from build123d import *

# Parameters (mm, degrees)
F1_DEPTH = 19.05
F2_R     = 76.2
F3_R     = 50.8
F4_R     = 8.994508
F5_DEPTH = 25.4


with BuildPart() as f1:
    # F0 (on Front) → F1 (new body)
    with BuildSketch(Plane.XZ):
        Polygon((-342.9, 69.85), (-342.9, 0), (266.7, 0), (266.7, 69.85), (139.7, 69.85), (58.081341, 127), (-58.081341, 127), (-139.7, 69.85), align=None)
    extrude(amount=F1_DEPTH)

    # F2
    f2_edges = [f1.edges().sort_by_distance(p)[0] for p in [
        (139.7, -9.525, 69.85),
        (58.081341, -9.525, 127),
        (-58.081341, -9.525, 127),
        (-139.7, -9.525, 69.85),
    ]]
    fillet(f2_edges, radius=F2_R)

    # F3
    f3_edges = [f1.edges().sort_by_distance(p)[0] for p in [
        (266.7, -9.525, 69.85),
        (-342.9, -9.525, 69.85),
    ]]
    fillet(f3_edges, radius=F3_R)

    # F4 (on face) → F5 (cut)
    with BuildSketch(Plane.XZ.offset(19.05)):
        with Locations((-292.1, 37.072986)):
            Circle(F4_R)
    extrude(amount=-F5_DEPTH, mode=Mode.SUBTRACT)


solid = f1.part
The model under review builds one solid part; all positions refer to its coordinate system, in mm. A direction names the side the tool comes from. Round coordinates to 2 decimals unless told otherwise and drop trailing zeros. Loops run counter-clockwise (first coordinate to the right, second up) from the corner with the lowest first, then second, coordinate; pieces in that order, holes last. Notation, with made-up numbers: (-6, 21) -> (28, 21) arc R10 cw to (28, 39) -> close; hole circle Ø3 at (-3.75, 79). An arc over 180 degrees is marked (long way). Write item = value, one per line. Start each with the question number.
Item 1: To check wall thickness, follow L1, parallel to Z at x = -292.1, y = -8.25; L2, parallel to Z at x = -178.5, y = -10.25; L3, parallel to X at y = -12, z = 25. State the ranges of each line that lie inside material, in increasing order.
Item 2: Take a section at B-B on x = -210. Give the boundary of the cut face in (y, z), plus the area to 3 significant figures.
Item 3: Take a section at A-A on y = -8.75. Give the boundary of the cut face in (x, z).
Item 4: Take a section at C-C on z = 89.5. Give the boundary of the cut face in (x, y), plus the area to 3 significant figures.
Item 5: Insertion check: pin 1 (9.5 mm diameter, centred on x = -214, y = -10, fed in from +Z); pin 2 (10 mm diameter, centred on y = -14, z = 28, fed in from -X); pin 3 (6 mm diameter, centred on y = -10, z = 81, fed in from +X); pin 4 (16 mm diameter, centred on x = -292.1, z = 37.07, fed in from +Y). Each pin has a flat end and moves straight along its axis. Give the tip position at first contact, or say it passes through.
Item 6: For faces 1 (the flat face through (-42, -19.05, 50)), 2 (the flat face through (190, -9, 69.85)), 3 (the flat face through (-227, -9, 69.85)), list the 3-axis set-ups (+Z, -Z, +X, -X, +Y, -Y) from which the entire face can be reached by the end or side of a thin tool; tool diameter is ignored.
Item 7: Mouldability with a two-part tool opening along X and no side actions: class faces 4 (the cylindrical face through (-301.086, -9.658, 37.468)), 5 (the flat face through (-98.595, -9.392, 98.632)), 6 (the flat face through (0, -9, 127)) as released by +X, released by -X, zero draft, split by the parting line, or undercut.
Result:
q1.L1 = 0 to 28.08, 46.07 to 69.85
q1.L2 = 0 to 69.85
q1.L3 = -342.55 to 266.35
q2.outline = (-19.05, 0) -> (0, 0) -> (0, 69.85) -> (-19.05, 69.85) -> close
q2.area = 1,330 mm²
q3.outline = (-342.9, 0) -> (266.7, 0) -> (266.7, 19.05) arc R50.8 ccw to (215.9, 69.85) -> (163.73, 69.85) arc R76.2 cw to (120.02, 83.63) -> (77.76, 113.22) arc R76.2 ccw to (34.06, 127) -> (-34.06, 127) arc R76.2 ccw to (-77.76, 113.22) -> (-120.02, 83.63) arc R76.2 cw to (-163.73, 69.85) -> (-292.1, 69.85) arc R50.8 ccw to (-342.9, 19.05) -> close; hole circle Ø17.99 at (-292.1, 37.07)
q4.outline = (-111.64, -19.05) -> (111.64, -19.05) -> (111.64, 0) -> (-111.64, 0) -> close
q4.area = 4,250 mm²
q5.pin_1 = 69.85
q5.pin_2 = -342.75
q5.pin_3 = 129.44
q5.pin_4 = through
q6.face_1 = +Z, -Z, +X, -X, -Y
q6.face_2 = +Z, +X, +Y, -Y
q6.face_3 = +Z, -X, +Y, -Y
q7.face_4 = undercut
q7.face_5 = released by -X
q7.face_6 = zero draft
